Autodesk Inventor part; units mm, degrees
ref_plane "YZ Plane" through (0, 0, 0) normal (1, 0, 0) x (0, 1, 0)
ref_plane "XZ Plane" through (0, 0, 0) normal (0, 1, 0) x (-1, 0, 0)
ref_plane "XY Plane" through (0, 0, 0) normal (0, 0, 1) x (1, 0, 0)
sketch "Sketch1" plane through (0, 0, 0) normal (0, 1, 0) x (-1, 0, 0)
  arc A0 (0, -5) -> (0, 5) centre (0, 0) ccw
  line L0 (0, 5) -> (0, -5)
  dimension "d0" = 10
extrude "Extrusion1" add sketch "Sketch1" along normal blind 10
sketch "Sketch2" plane through (0, 0, 0) normal (1, 0, 0) x (0, 1, 0)
  line L0 (8.0172, -4.5) -> (8.0172, 4.5)
  line L1 (8.0172, 4.5) -> (2.5172, 4.5)
  line L2 (2.5172, -4.5) -> (0.0172, -2)
  line L3 (2.5172, 4.5) -> (0.0172, 2)
  line L4 (0.0172, -2) -> (0.0172, 2)
  line L5 (8.0172, -4.5) -> (2.5172, -4.5)
  point P0 (0, 0)
  dimension "d3" = 9
  dimension "d4" = 8
sketch "Sketch3" plane through (0, 0, 0) normal (1, 0, 0) x (0, 1, 0)
  line L0 (0, 2) -> (3, 5)
  arc A0 (3, 5) -> (0, 2) centre (1, 4) ccw
  line L1 (0, -2) -> (4, -6)
  arc A1 (0, -2) -> (4, -6) centre (1.75, -4.25) ccw
  line L2 (8.0325, 5) -> (11, 5)
  line L3 (11, 5) -> (11, -6)
  line L4 (11, -6) -> (8.0325, -6)
  line L5 (8.0325, -6) -> (8.0325, 5)
  line L6 (2.4911, 4.4911) -> (5, 7)
  line L7 (2.4911, 4.4911) -> (8.0325, 4.4911)
  arc A2 (8.0325, 4.4911) -> (5, 7) centre (7, 6.3303) ccw
  line L8 (2.4911, -4.4911) -> (8.5706, -4.4911)
  arc A3 (2.4911, -4.4911) -> (8.5706, -4.4911) centre (5.5309, -7.5041) ccw
  point P0 (0, 0)
extrude "Extrusion2" cut sketch "Sketch3" against normal through all
sketch "Sketch4" plane through (0, 0, 0) normal (0, 1, 0) x (-1, 0, 0)
  arc A0 (1.0726, -4.4911) -> (1.0726, 4.4911) centre (-1.125, 0) ccw
  arc A1 (1.0726, 4.4911) -> (1.0726, -4.4911) centre (-0.4517, 0) ccw
  point P0 (0, 0)
  point P1 (2.1976, -4.4911)
  point P2 (2.1976, 4.4911)
  dimension "d9" = 1.125
  dimension "d10" = 1.125
extrude "Extrusion3" cut sketch "Sketch4" along normal through all both and the other way through all
sketch "Sketch5" plane through (0, 0, 0) normal (1, 0, 0) x (0, 1, 0)
  line L0 (1.6, -1.2445) -> (1.6, 1.1555)
  line L1 (6.4325, 2.6911) -> (3.1125, 2.6911)
  line L2 (6.4325, -2.6911) -> (6.4325, 2.6911)
  line L3 (6.4325, -2.6911) -> (3.1125, -2.6911)
  line L4 (0, 2) -> (0, -2)
  line L5 (8.0325, 4.4911) -> (8.0325, -4.4911)
  line L6 (0, 2) -> (2.4911, 4.4911)
  line L7 (2.4911, 4.4911) -> (8.0325, 4.4911)
  line L8 (8.0325, 4.4911) -> (8.0325, -4.4911)
  line L9 (8.0325, -4.4911) -> (2.4911, -4.4911)
  line L10 (2.4911, -4.4911) -> (0, -2)
  line L11 (0, 2) -> (0, -2)
  line L12 (1.6, 1.1555) -> (3.1125, 2.6911)
  line L13 (1.6, -1.2445) -> (3.1125, -2.6911)
  line L14 (1.6, 4.6579) -> (1.6, -5.3823)
  arc A0 (1.6, 4.6579) -> (1.6, -5.3823) centre (3.2437, -0.3622) ccw
  line L15 (1.6, 1.1555) -> (5.4757, 5.0906)
  line L16 (1.6, 1.1555) -> (1.6, 7.5999)
  arc A1 (5.4757, 5.0906) -> (1.6, 7.5999) centre (3.8837, 6.8794) ccw
  line L17 (3.1125, 2.6911) -> (12.4034, 2.6911)
  line L18 (3.1125, 2.6911) -> (8.5318, 8.1936)
  arc A2 (12.4034, 2.6911) -> (8.5318, 8.1936) centre (8.3272, 3.9364) ccw
  line L19 (6.4325, 2.6911) -> (13.6333, 2.6911)
  line L20 (6.4325, 2.6911) -> (6.4325, -9.3636)
  arc A3 (6.4325, -9.3636) -> (13.6333, 2.6911) centre (6.37, -1.1482) ccw
  line L21 (6.4325, -2.6911) -> (6.4325, -11.5775)
  line L22 (6.4325, -2.6911) -> (3.1125, -2.6911)
  line L23 (3.1125, -2.6911) -> (3.2437, -12.8567)
  arc A4 (3.2437, -12.8567) -> (6.4325, -9.3636) centre (5.6123, -11.8169) ccw
  line L24 (1.6, -1.2445) -> (1.6, -8.2222)
  line L25 (1.6, -1.2445) -> (3.1125, -2.6911)
  line L26 (3.1125, -2.6911) -> (3.1946, -9.0574)
  arc A5 (1.6, -8.2222) -> (3.1946, -9.0574) centre (2.6381, -8.1801) ccw
  point P0 (0, 0)
  dimension "d16" = 1.6
  dimension "d18" = 1.6
  dimension "d21" = 1.8
  dimension "d23" = 1.8
  dimension "d24" = 2.4
  dimension "d26" = 3.32
  dimension "d27" = 3.32
extrude "Extrusion4" cut sketch "Sketch5" against normal through all contours L14 L10 L4 L6 L0 | L13 L23 L9 L10 L14 | L14 L6 L7 L15 L12 | L3 L20 L9 L23 | L14 A0 L6 L4 L10 | L10 L9 L23 A5 L24 L14 | L15 L7 L5 L17 L1 | L14 L16 A1 L15 L7 L6 | L2 L17 L5 L9 L20 | L9 L20 A4 L23 | L15 L18 A2 L17 L5 L7 | L9 L5 L17 L19 A3 L20
sketch "Sketch6" plane through (0, 0, 0) normal (1, 0, 0) x (0, 1, 0)
  circle A0 centre (4, 0) radius 1.575
  line L0 (1.6, -1.2445) -> (1.6, 1.1555)
  point P0 (0, 0)
  dimension "d31" = 3.15
  dimension "d32" = 2.4
extrude "Extrusion5" add sketch "Sketch6" against normal blind 15
sketch "Sketch7" plane through (0, 0, 0) normal (0, 1, 0) x (-1, 0, 0)
  arc A0 (3.089, -2.6911) -> (3.7176, -1.2445) centre (-1.125, 0) ccw
  arc A1 (3.7397, 1.1555) -> (3.089, 2.6911) centre (-1.125, 0) ccw
  arc A2 (3.7176, -1.2445) -> (3.7397, 1.1555) centre (-1.125, 0) ccw
  arc A3 (3.089, 2.6911) -> (3.089, -2.6911) centre (1.8078, 0) ccw
  point P0 (0, 0)
extrude "Extrusion6" cut sketch "Sketch7" along normal through all
sketch "Sketch8" plane through (-15, 4, 0) normal (-1, 0, 0) x (0, 0, 1)
  circle A0 centre (0, 0) radius 0.5375
  point P0 (0, -4)
  dimension "d37" = 1.075
extrude "Extrusion7" cut sketch "Sketch8" against normal blind 10
properties part number "10mm_radius_labmaker_cSkull_mold_window_stabilizer_Apr0119"
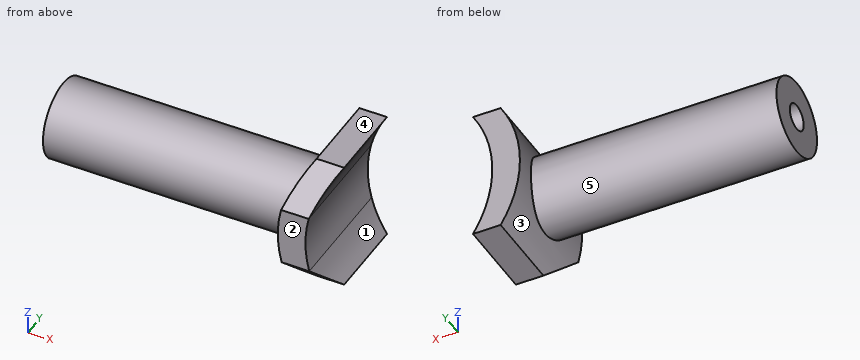
For this review, take the finished solid that the model builds, in its own axes (mm). Face numbers are marked on the shaded views. A direction names the side the tool comes from. Round coordinates to 2 decimals unless told otherwise and drop trailing zeros. Order: outer loops, then holes, each group sorted by start corner. A loop starts at its lowest first (then second) coordinate and runs counter-clockwise, first axis right, second up.
Q1. Wall thickness on line 1 (Y direction, x = -6.75, z = 0) (1 decimal); line 2 (X direction, y = 4.4, z = -1.25); line 3 (X direction, y = 3.95, z = 2.15): over which ranges is each line inside the solid? List them lowest first.
Findings below:
line 1: y = 2.4 to 3.5, 4.5 to 5.6
line 2: x = -15 to -3.72
line 3: x = -4.51 to -3.39
Q2. Mouldability with a two-part tool opening along Z and no side actions: class the marked faces 1, 2 and 3 as pulls with the +Z half, pulls with the -Z half, needs draft (parallel to the pull), parting line crosses it, or undercut.
Findings below:
face 1: undercut
face 2: needs draft
face 3: parting line crosses it
Q3. We need section D-D, the plane y = 5.1. Give the boundary of the cut face in (x, z).
Findings below:
outline: (-15, -1.13) - (-4.87, -1.13) arc R5 ccw to (-4.21, -2.69) - (-3.09, -2.69) arc R5 cw to (-3.72, -1.24) arc R5 cw to (-3.74, 1.16) arc R5 cw to (-3.09, 2.69) - (-4.21, 2.69) arc R5 ccw to (-4.87, 1.13) - (-15, 1.13) - close
Q4. Machinability: for the marked faces 4 and 5, which of the approach directions +Z, -Z, +X, -X, +Y, -Y give a long, thin tool a straight path to every point of the face, cutting with its end or side? Answer none if there is none.
Findings below:
face 4: +Z, +X, -X, +Y, -Y
face 5: -X
Q5. We need section B-B, the plane z = 0. Give the boundary of the cut face in (x, y) (1 decimal).
Findings below:
outline: (-15, 2.4) - (-5, 2.4) - (-5, 1.6) - (-3.9, 1.6) - (-3.9, 6.4) - (-5, 6.4) - (-5, 5.6) - (-15, 5.6) - (-15, 4.5) - (-5, 4.5) - (-5, 3.5) - (-15, 3.5) - close
Q6. Insertion check: P1, Ø0.5, axis at y = 4, z = 0, coming from the -X side; P2, Ø1.4, axis at y = 4, z = 0, coming from the +X side. Each pin has a flat end and moves straight along its axis. Give the tip position at first contact, or say it passes through.
Findings below:
P1: stops at x = -5
P2: stops at x = -3.83
Q7. We need section A-A, the plane y = 4. Give the boundary of the cut face in (x, z) (1 decimal).
Findings below:
outline: (-15, -1.6) - (-4.7, -1.6) arc R5 ccw to (-4.2, -2.7) - (-3.1, -2.7) arc R5 cw to (-3.7, -1.2) arc R5 cw to (-3.7, 1.2) arc R5 cw to (-3.1, 2.7) - (-4.2, 2.7) arc R5 ccw to (-4.7, 1.6) - (-15, 1.6) - (-15, 0.5) - (-5, 0.5) - (-5, -0.5) - (-15, -0.5) - close
